For this review, take the finished solid that the model builds, in its own axes (mm). Face numbers are marked on the shaded views. Give positions to 0.01 mm unless a question says otherwise; leave off trailing zeros. Order: outer loops, then holes, each group sorted by start corner. A loop starts at its lowest first (then second) coordinate and runs counter-clockwise, first axis right, second up.
Item 1: Consider section C-C (y = 8.75). Give the boundary of the cut face in (x, z).
Item 2: For probe 1 along Z at (x, y) = (0, 14.5); probe 2 along Z at (x, y) = (0, 8.5); probe 3 along Y at (x, z) = (-5.5, -11), list the stretches that pass through material, from the lowest coordinate up.
Item 3: The part is to be moulded in two halves that separate along Z. For the marked faces 1, 2 and 3, say which applies: released by +Z, released by -Z, zero draft, split by the parting line, or undercut.
Item 4: For P1, Ø1, axis at y = 1, z = -29.5, coming from the -X side; P2, Ø3, axis at x = 5.5, z = 19.5, coming from the +Y side; P3, Ø8, axis at x = 24, y = 13.5, coming from the -Z side, all flat-tipped, find the tip position at first contact; note any pin that passes through.
Item 5: Consider section A-A (x = -28.5). Give the boundary of the cut face in (y, z).
Item 6: Consider section B-B (z = 0). Give the boundary of the cut face in (x, y), plus the area to 3 significant figures.
Autodesk Inventor part; units mm, degrees
ref_plane "YZ Plane" through (0, 0, 0) normal (1, 0, 0) x (0, 1, 0)
ref_plane "XZ Plane" through (0, 0, 0) normal (0, 1, 0) x (-1, 0, 0)
ref_plane "XY Plane" through (0, 0, 0) normal (0, 0, 1) x (1, 0, 0)
sketch "Sketch4" plane through (0, 0, 0) normal (0, 1, 0) x (-1, 0, 0)
  circle A0 centre (0, 0) radius 39.75
  circle A1 centre (0, 0) radius 41.6215
  circle A2 centre (0, 0) radius 41.6213
  dimension "d17" = 79.5
  dimension "d18" = 83.243
sketch "Sketch6" plane through (0, 0, 0) normal (0, 1, 0) x (-1, 0, 0)
  circle A0 centre (0, 0) radius 39.7618
extrude "Extrusion1" add sketch "Sketch6" along normal blind 3
extrude "Extrusion2" add sketch "Sketch4" along normal blind 13
sketch "Sketch7" plane through (0, 0, 0) normal (0, -1, 0) x (1, 0, 0)
  circle A0 centre (0, 0) radius 44.86
  circle A1 centre (0, 0) radius 41.6213
extrude "Extrusion3" add sketch "Sketch7" against normal blind 18
sketch "Sketch8" plane through (0, 0, 0) normal (0, -1, 0) x (1, 0, 0)
  circle A0 centre (0, 0) radius 44.86
extrude "Extrusion4" add sketch "Sketch8" along normal blind 1
properties part number "Soft Coating Gripper mold_10mil"
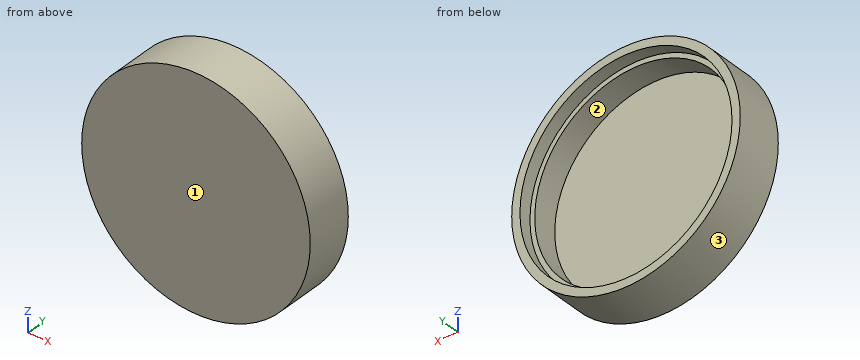
Resolved:
1. outline: circle Ø89.72 at (0, 0); hole circle Ø79.5 at (0, 0)
2. probe 1: z = -44.86 to -41.62, 41.62 to 44.86
2. probe 2: z = -44.86 to -39.75, 39.75 to 44.86
2. probe 3: y = -1 to 3
3. face 1: zero draft
3. face 2: undercut
3. face 3: split by the parting line
4. P1: stops at x = -34.23
4. P2: stops at y = 3
4. P3: stops at z = -40.15
5. outline: (-1, -34.64) - (18, -34.64) - (18, -30.33) - (13, -30.33) - (13, -27.71) - (3, -27.71) - (3, 27.71) - (13, 27.71) - (13, 30.33) - (18, 30.33) - (18, 34.64) - (-1, 34.64) - close
6. outline: (-44.86, -1) - (44.86, -1) - (44.86, 18) - (41.62, 18) - (41.62, 13) - (39.75, 13) - (39.75, 3) - (-39.75, 3) - (-39.75, 13) - (-41.62, 13) - (-41.62, 18) - (-44.86, 18) - close
6. area: 493 mm2
